from build123d import *

# Parameters (mm, degrees)
ESQUISSE11_R        = 3.75
ESQUISSE11_R_2      = 1.5
BOSS_EXTRU_11_DEPTH = 3


with BuildPart() as part:
    # Esquisse11 → Boss.-Extru.11 (new body)
    with BuildSketch(Plane.XY):
        Polygon((-66.008134961, -86.49661352), (-66.008134961, -75.49661352), (-69.008134961, -75.49661352), (-69.008134961, -65.49661352), (-19.008134961, -65.49661352), (-19.008134961, -75.49661352), (-22.008134961, -75.49661352), (-22.008134961, -86.49661352), (-26.008134961, -86.49661352), (-26.008134961, -84.99661352), (-28.508134961, -84.99661352), (-28.508134961, -86.49661352), (-32.008134961, -86.49661352), (-32.008134961, -89.49661352), (-28.508134961, -89.49661352), (-28.508134961, -90.99661352), (-26.008134961, -90.99661352), (-26.008134961, -89.49661352), (-22.008134961, -89.49661352), (-22.008134961, -100.49661352), (-19.008134961, -100.49661352), (-19.008134961, -110.49661352), (-69.008134961, -110.49661352), (-69.008134961, -100.49661352), (-66.008134961, -100.49661352), (-66.008134961, -89.49661352), (-62.008134961, -89.49661352), (-62.008134961, -90.99661352), (-59.508134961, -90.99661352), (-59.508134961, -89.49661352), (-56.008134961, -89.49661352), (-56.008134961, -86.49661352), (-59.508134961, -86.49661352), (-59.508134961, -84.99661352), (-62.008134961, -84.99661352), (-62.008134961, -86.49661352), align=None)
        with Locations((-44.008134961, -88.045619642)):
            Circle(ESQUISSE11_R, mode=Mode.SUBTRACT)
        with Locations((-37.008134961, -88.045619642)):
            Circle(ESQUISSE11_R_2, mode=Mode.SUBTRACT)
        with Locations((-51.008134961, -88.045619642)):
            Circle(ESQUISSE11_R_2, mode=Mode.SUBTRACT)
        with Locations((-44.008134961, -77.045619642)):
            Circle(ESQUISSE11_R_2, mode=Mode.SUBTRACT)
        with Locations((-44.008134961, -99.045619642)):
            Circle(ESQUISSE11_R_2, mode=Mode.SUBTRACT)
        with Locations((-41.008134961, -68.99661352)):
            Circle(ESQUISSE11_R_2, mode=Mode.SUBTRACT)
        with Locations((-41.008134961, -106.99661352)):
            Circle(ESQUISSE11_R_2, mode=Mode.SUBTRACT)
    extrude(amount=BOSS_EXTRU_11_DEPTH)


solid = part.part
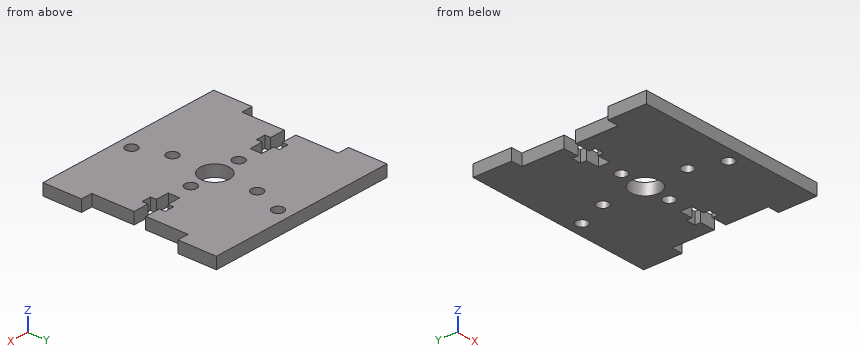
Build history of the part. All positions in model axes, mm. Coordinates: 2 decimals unless noted, no trailing zeros. Order: outer loops, then holes, each group sorted by start corner. A loop starts at its lowest first (then second) coordinate and runs counter-clockwise, first axis right, second up. Notation, with made-up numbers: (39.25, 62) - (66.25, 62) arc R30 ccw to (66.25, 98) - close; hole circle Ø9 at (21.25, 58.25). An arc over 180 degrees is marked (long way). Write each question's results on one line, items separated by ' | '. Start each with the question number.
Item 1: Flat gauge pins, fed straight in: pin 1 (10 mm diameter, centred on x = -44, y = -90.5, fed in from -Z); pin 2 (1.6 mm diameter, centred on y = -90.5, z = 1, fed in from +X). Where does each tip first touch, or does it go through?
Item 2: Band-saw the part on D-D on z = 1.65. State how many separate pieces and enclosed holes the cut face has, and give its area (3 significant figures).
Item 3: Band-saw the part on A-A on x = -65. Write the cut outline in (y, z), and give its area (3 significant figures).
Item 4: Band-saw the part on B-B on x = -37.5. Write the cut outline in (y, z).
Item 5: Band-saw the part on C-C on y = -96.5. Write the cut outline in (x, z), and give its area (3 significant figures).
Item 6: Wall check: probe 1 along Y at (x, z) = (-58, 2.05); probe 2 along Y at (x, z) = (-28, 1); probe 3 along Y at (x, z) = (-43, 2.45). Give the ranges that are in metal, low to high. Write a range as [from, to].
Numbers:
1) pin 1: z = 0 | pin 2: x = -22.01
2) separate pieces: 1 | enclosed holes: 7 | area: 1,940 mm^2
3) outline: (-110.5, 0) - (-89.5, 0) - (-89.5, 3) - (-110.5, 3) - close; (-86.5, 0) - (-65.5, 0) - (-65.5, 3) - (-86.5, 3) - close | area: 126 mm^2
4) outline: (-110.5, 0) - (-89.46, 0) - (-89.46, 3) - (-110.5, 3) - close; (-86.63, 0) - (-65.5, 0) - (-65.5, 3) - (-86.63, 3) - close
5) outline: (-66.01, 0) - (-22.01, 0) - (-22.01, 3) - (-66.01, 3) - close | area: 132 mm^2
6) probe 1: [-110.5, -89.5], [-86.5, -65.5] | probe 2: [-110.5, -91], [-85, -65.5] | probe 3: [-110.5, -100.16], [-97.93, -91.66], [-84.43, -78.16], [-75.93, -65.5]
